```python
from build123d import *

# Parameters (mm, degrees)
SKETCH_R     = 2.5
SKETCH_R_2   = 5
PAD_DEPTH    = 5
CHAMFER_SIZE = 4


with BuildPart() as part:
    # Sketch → Pad (new body)
    with BuildSketch(Plane.XY):
        Polygon((84, 110.25), (44, 110.25), (0, 53.75), (0, 0), (84, 0), align=None)
        with Locations((15, 45.25)):
            Circle(SKETCH_R, mode=Mode.SUBTRACT)
        with Locations((15, 12.25)):
            Circle(SKETCH_R, mode=Mode.SUBTRACT)
        with Locations((15, 28.75)):
            Circle(SKETCH_R_2, mode=Mode.SUBTRACT)
        with Locations((53, 47)):
            Circle(SKETCH_R, mode=Mode.SUBTRACT)
        with Locations((53, 28.75)):
            Circle(SKETCH_R_2, mode=Mode.SUBTRACT)
        with Locations((53, 10.5)):
            Circle(SKETCH_R, mode=Mode.SUBTRACT)
        with Locations((54, 80.25)):
            Circle(SKETCH_R, mode=Mode.SUBTRACT)
        with Locations((74, 80.25)):
            Circle(SKETCH_R, mode=Mode.SUBTRACT)
        with Locations((54, 100.25)):
            Circle(SKETCH_R, mode=Mode.SUBTRACT)
        with Locations((74, 100.25)):
            Circle(SKETCH_R, mode=Mode.SUBTRACT)
    extrude(amount=PAD_DEPTH)

    # Chamfer
    chamfer_edges = [part.edges().sort_by_distance(p)[0] for p in [
        (0, 0, 2.5),
        (84, 0, 2.5),
    ]]
    chamfer(chamfer_edges, length=CHAMFER_SIZE)


solid = part.part
```
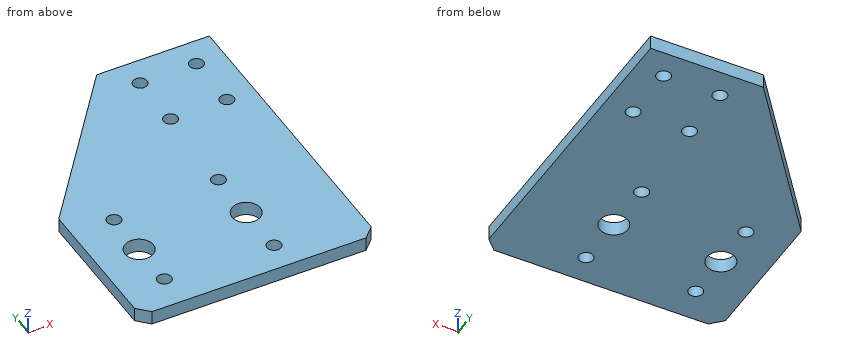
Geometry: final body of the model. Coordinates: model frame, mm. Coordinates: 2 decimals unless noted, no trailing zeros. Order: outer loops, then holes, each group sorted by start corner. A loop starts at its lowest first (then second) coordinate and runs counter-clockwise, first axis right, second up.
Item 1: Section query A-A (z = 1.9). State how many separate pieces and enclosed holes the cut face has, then the cut area to 3 significant figures.
Answer:
separate pieces: 1
enclosed holes: 10
area: 7,690 mm2
Item 2: Material intervals for line 1 along Y through (x, z) = (74, 1.1); line 2 along Y through (x, z) = (54, 2.2); line 3 along X through (y, z) = (78, 2.6), sorted ascending.
Answer:
line 1: y = 0 to 77.75, 82.75 to 97.75, 102.75 to 110.25
line 2: y = 0 to 8.21, 12.79 to 23.85, 33.65 to 44.71, 49.29 to 77.75, 82.75 to 97.75, 102.75 to 110.25
line 3: x = 18.88 to 52.91, 55.09 to 72.91, 75.09 to 84
Item 3: Section query D-D (y = 65). Output: boundary loops of the cut face in (x, z), then the cut area to 3 significant figures.
Answer:
outline: (8.76, 0) - (84, 0) - (84, 5) - (8.76, 5) - close
area: 376 mm2
Item 4: Section query B-B (y = 28.75). Output: boundary loops of the cut face in (x, z).
Answer:
outline: (0, 0) - (10, 0) - (10, 5) - (0, 5) - close; (20, 0) - (48, 0) - (48, 5) - (20, 5) - close; (58, 0) - (84, 0) - (84, 5) - (58, 5) - close
Item 5: Section query C-C (x = 74). Output: boundary loops of the cut face in (y, z), then the cut area to 3 significant figures.
Answer:
outline: (0, 0) - (77.75, 0) - (77.75, 5) - (0, 5) - close; (82.75, 0) - (97.75, 0) - (97.75, 5) - (82.75, 5) - close; (102.75, 0) - (110.25, 0) - (110.25, 5) - (102.75, 5) - close
area: 501 mm2
Item 6: Contact query for a flat-ended pin moving along its axis: P1, Ø3, axis at x = 53, y = 10.5, coming from the -Z side. Output: stop coordinate, or through.
Answer:
P1: passes through
